Job drawing, mm, ordinate dimensions from the low corner. One solid piece. Round coordinates to 2 decimals unless told otherwise and drop trailing zeros. Order: outer loops, then holes, each group sorted by start corner. A loop starts at its lowest first (then second) coordinate and runs counter-clockwise, first axis right, second up. Notation, with made-up numbers: (63.5, 0) -> (109.5, 0) arc R9 ccw to (109.5, 16) -> close; hole circle Ø2 at (23, 5). An arc over 180 degrees is marked (long way). Return JSON: item names as keys, results as strings. Group by question number.
Q1. Cut at B-B (x = 5). Write the cut outline in (y, z), then the cut area to 3 significant figures.
Q2. Cut at C-C (y = 30). Write the cut outline in (x, z).
Q3. Cut at D-D (z = 1.5). Write the cut outline in (x, y), then the cut area to 3 significant figures.
Q4. Cut at A-A (z = 5). Write the cut outline in (x, y).
Q5. Probe line 1 along Z through (x, y) = (6, 30); line 2 along Y through (x, z) = (3.25, 6.25); line 3 along Y through (x, z) = (8, 6.75). List the from-to ranges inside material, lowest first.
Q6. Mould opens along Y. For the marked faces 1, 2, 3 and 4 say: +Y half, -Y half, draft (parallel to the pull), parting line (faces both ways), or undercut.
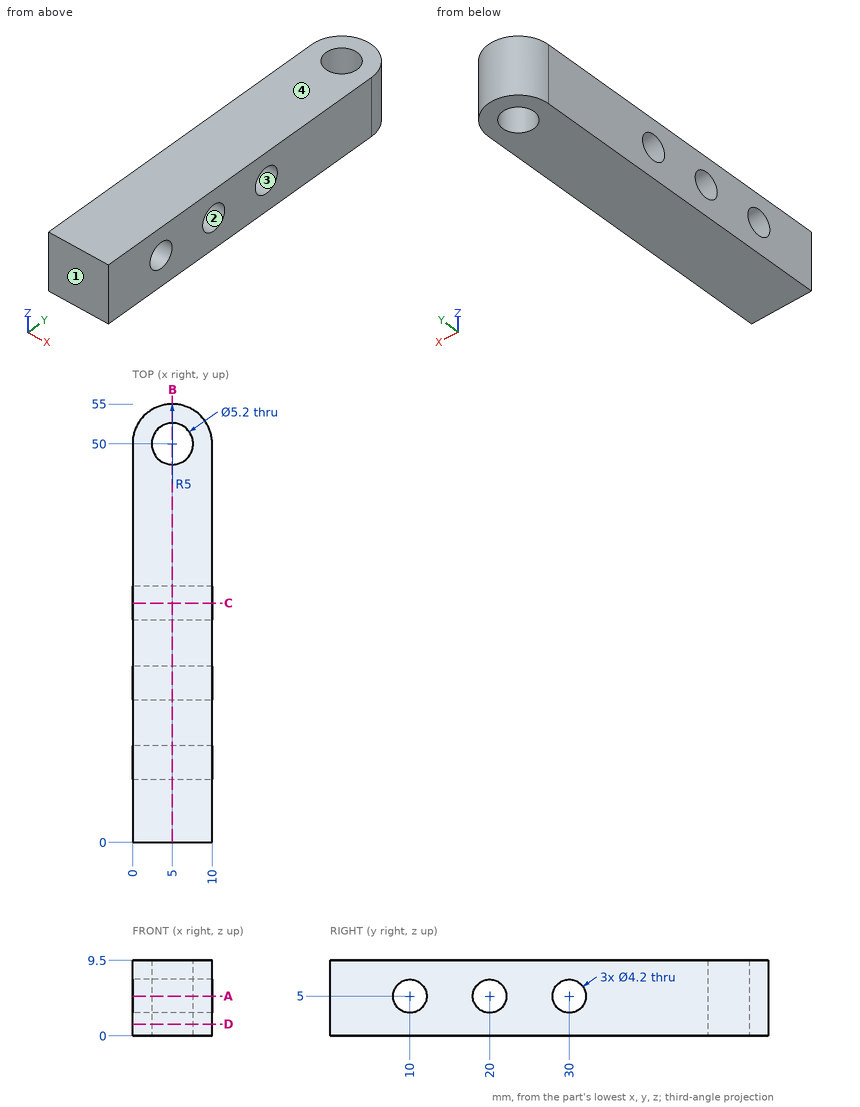
Solution:
{
 "1": {"outline": "(0, 0) -> (47.4, 0) -> (47.4, 9.5) -> (0, 9.5) -> close; (52.6, 0) -> (55, 0) -> (55, 9.5) -> (52.6, 9.5) -> close; hole circle Ø4.2 at (10, 5); hole circle Ø4.2 at (20, 5); hole circle Ø4.2 at (30, 5)", "area": "432 mm²"},
 "2": {"outline": "(0, 0) -> (10, 0) -> (10, 2.9) -> (0, 2.9) -> close; (0, 7.1) -> (10, 7.1) -> (10, 9.5) -> (0, 9.5) -> close"},
 "3": {"outline": "(0, 0) -> (10, 0) -> (10, 50) arc R5 ccw to (0, 50) -> close; hole circle Ø5.2 at (5, 50)", "area": "518 mm²"},
 "4": {"outline": "(0, 0) -> (10, 0) -> (10, 7.9) -> (0, 7.9) -> close; (0, 12.1) -> (10, 12.1) -> (10, 17.9) -> (0, 17.9) -> close; (0, 22.1) -> (10, 22.1) -> (10, 27.9) -> (0, 27.9) -> close; (0, 32.1) -> (10, 32.1) -> (10, 50) arc R5 ccw to (0, 50) -> close; hole circle Ø5.2 at (5, 50)"},
 "5": {"line 1": "z = 0 to 2.9, 7.1 to 9.5", "line 2": "y = 0 to 8.31, 11.69 to 18.31, 21.69 to 28.31, 31.69 to 48.08, 51.92 to 54.68", "line 3": "y = 0 to 8.84, 11.16 to 18.84, 21.16 to 28.84, 31.16 to 54"},
 "6": {"face 1": "-Y half", "face 2": "undercut", "face 3": "undercut", "face 4": "draft"}
}
